from build123d import *

# Parameters (mm, degrees)
F1_DEPTH = 101.6
F2_DEPTH = 25.4


with BuildPart() as f1:
    # F0 (on Front) → F1 (new body)
    with BuildSketch(Plane.XZ):
        Polygon((-41.275, -9.525), (41.275, -9.525), (41.275, 9.525), (22.225, 9.525), (-41.275, 9.525), align=None)
    extrude(amount=F1_DEPTH)

    # F0 (on Front) → F2 (join)
    with BuildSketch(Plane.XZ):
        Polygon((-41.275, -9.525), (41.275, -9.525), (41.275, 9.525), (22.225, 9.525), (-41.275, 9.525), align=None)
        with BuildLine():
            Line((22.225, 9.525), (41.275, 9.525))
            Line((41.275, 9.525), (41.275, 37.5267544395))
            ThreePointArc((41.275, 37.5267544395), (45.9246798487, 48.7520745908), (57.15, 53.4017544395))
            Line((57.15, 53.4017544395), (62.2553965644, 53.4017544395))
            Line((62.2553965644, 53.4017544395), (62.2553965644, 71.7100659957))
            add(Edge.make_bspline(
                [(61.1839862246, 72.4517544395), (61.5444478672, 72.2168104336), (61.9016010693, 71.9696416328), (62.2553965644, 71.7100659957)],
                knots=[0.5333237342, 0.5333237342, 0.5333237342, 0.5333237342, 0.5412655487, 0.5412655487, 0.5412655487, 0.5412655487], degree=3))
            Line((61.1839862246, 72.4517544395), (57.15, 72.4517544395))
            ThreePointArc((57.15, 72.4517544395), (32.4542956671, 62.2224587724), (22.225, 37.5267544395))
            Line((22.225, 37.5267544395), (22.225, 9.525))
        make_face()
        with BuildLine():
            add(Edge.make_bspline(
                [(-41.275, 9.525), (-2.1487074739, 48.87707908), (36.9775850521, 88.2291581599), (61.1839862246, 72.4517544395)],
                knots=[0, 0, 0, 0, 0.5333237342, 0.5333237342, 0.5333237342, 0.5333237342], degree=3))
            Line((-41.275, 9.525), (22.225, 9.525))
            Line((22.225, 9.525), (22.225, 37.5267544395))
            ThreePointArc((22.225, 37.5267544395), (32.4542956671, 62.2224587724), (57.15, 72.4517544395))
            Line((57.15, 72.4517544395), (61.1839862246, 72.4517544395))
        make_face()
        with BuildLine():
            Line((87.63, 72.4517544395), (61.1839862246, 72.4517544395))
            add(Edge.make_bspline(
                [(61.1839862246, 72.4517544395), (61.5444478672, 72.2168104336), (61.9016010693, 71.9696416328), (62.2553965644, 71.7100659957)],
                knots=[0.5333237342, 0.5333237342, 0.5333237342, 0.5333237342, 0.5412655487, 0.5412655487, 0.5412655487, 0.5412655487], degree=3))
            Line((62.2553965644, 71.7100659957), (87.63, 71.7100659957))
            Line((87.63, 71.7100659957), (87.63, 72.4517544395))
        make_face()
        with BuildLine():
            add(Edge.make_bspline(
                [(62.2553965644, 71.7100659957), (67.5956887588, 67.7919557655), (72.1709689679, 61.0471014204), (75.9112780576, 53.4017544395)],
                knots=[0.5412655487, 0.5412655487, 0.5412655487, 0.5412655487, 0.6611416096, 0.6611416096, 0.6611416096, 0.6611416096], degree=3))
            Line((62.2553965644, 71.7100659957), (62.2553965644, 53.4017544395))
            Line((62.2553965644, 53.4017544395), (75.9112780576, 53.4017544395))
        make_face()
        with BuildLine():
            Line((87.63, 71.7100659957), (62.2553965644, 71.7100659957))
            add(Edge.make_bspline(
                [(62.2553965644, 71.7100659957), (67.5956887588, 67.7919557655), (72.1709689679, 61.0471014204), (75.9112780576, 53.4017544395)],
                knots=[0.5412655487, 0.5412655487, 0.5412655487, 0.5412655487, 0.6611416096, 0.6611416096, 0.6611416096, 0.6611416096], degree=3))
            Line((75.9112780576, 53.4017544395), (87.63, 53.4017544395))
            Line((87.63, 53.4017544395), (87.63, 71.7100659957))
        make_face()
        with BuildLine():
            Line((75.9112780576, 53.4017544395), (62.2553965644, 53.4017544395))
            Line((62.2553965644, 53.4017544395), (62.2553965644, 43.1350659957))
            Line((62.2553965644, 43.1350659957), (80.2891256511, 43.1350659957))
            add(Edge.make_bspline(
                [(75.9112780576, 53.4017544395), (77.5285535174, 50.0959762919), (78.989721228, 46.6218403707), (80.2891256511, 43.1350659957)],
                knots=[0.6611416096, 0.6611416096, 0.6611416096, 0.6611416096, 0.7129749225, 0.7129749225, 0.7129749225, 0.7129749225], degree=3))
        make_face()
        Polygon((113.0553965644, 71.7100659957), (87.63, 71.7100659957), (87.63, 53.4017544395), (87.63, 43.1350659957), (113.0553965644, 43.1350659957), align=None)
        with BuildLine():
            Line((87.63, 53.4017544395), (75.9112780576, 53.4017544395))
            add(Edge.make_bspline(
                [(75.9112780576, 53.4017544395), (77.5285535174, 50.0959762919), (78.989721228, 46.6218403707), (80.2891256511, 43.1350659957)],
                knots=[0.6611416096, 0.6611416096, 0.6611416096, 0.6611416096, 0.7129749225, 0.7129749225, 0.7129749225, 0.7129749225], degree=3))
            Line((80.2891256511, 43.1350659957), (87.63, 43.1350659957))
            Line((87.63, 43.1350659957), (87.63, 53.4017544395))
        make_face()
    extrude(amount=F2_DEPTH)


solid = f1.part
Geometry check sheet. Reference: the model listing, model coordinates, mm. A direction names the side the tool comes from. Give positions to 0.01 mm unless a question says otherwise; leave off trailing zeros. Write each loop counter-clockwise with the first axis right and the second up, starting at its lowest first coordinate (ties: lowest second). Pieces come first, ordered by that corner, then holes. Notation, with made-up numbers: M -27.5,-14 L 11.5,-14 A29 cw 11.5,17 Z; hole C 1.5,25 d4. An arc over 180 degrees is marked long. One line per question, with ' | ' between items.
1. Cross-section at B-B (x = 69). Enter the section's corners in (y, z).
Ans:
outline: M -25.4,43.14 L 0,43.14 L 0,72.45 L -25.4,72.45 Z
2. Cross-section at A-A (z = 6). Enter the section's corners in (x, y) (3 decimals).
Ans:
outline: M -41.275,-101.6 L 41.275,-101.6 L 41.275,0 L -41.275,0 Z
3. Gauge pin test, flat ends, axial feed: pin 1 (8 mm diameter, centred on x = 37.5, y = -37.5, fed in from +Z) (3 decimals); pin 2 (8 mm diameter, centred on y = -18, z = 49, fed in from -X); pin 3 (4 mm diameter, centred on x = 6, z = 27, fed in from -Y). Record the tip position at first contact, or that the pin passes through.
Ans:
pin 1: z = 9.525 | pin 2: x = -4.76 | pin 3: y = -25.4
4. Mould release check, pull along X, two halves, no side actions. Record for faces 1 (the face through (45.802, -12.522, 48.628)), 2 (the face through (-41.275, -50, 0)), 3 (the face through (35, -25.4, 41)), 4 (the face through (62.255, -13, 48)): released by +X, released by -X, zero draft, split by the parting line, or undercut.
Ans:
face 1: undercut | face 2: released by -X | face 3: zero draft | face 4: undercut
5. Scan lines: line 1 along Y through (x, z) = (15.5, 35); line 2 along Z through (x, y) = (-33.5, -30) (3 decimals); line 3 along Z through (x, y) = (103.5, -7). Record each from-to range of solid material in increasing order. Write a range as from..to.
Ans:
line 1: -25.4..0 | line 2: -9.525..9.525 | line 3: 43.14..71.71
6. Set-up check for faces 5 (the face through (1, -63, 9.525)), 6 (the face through (87, -13, 43.135)), 7 (the face through (-1, -50, -9.525)), 8 (the face through (60, -13, 53.402)), 9 (the face through (101, -13, 71.71)): record each of +Z, -Z, +X, -X, +Y, -Y from which the full face is reachable in a straight line by a thin tool's end or side.
Ans:
face 5: +Z, +X, -X, -Y | face 6: -Z, +X, +Y, -Y | face 7: -Z, +X, -X, +Y, -Y | face 8: -Z, +Y, -Y | face 9: +Z, +X, +Y, -Y
